```python
from build123d import *

# Parameters (mm, degrees)
PIN_DRAWING_W       = 0.636
PIN_DRAWING_H       = 0.636
BOSS_EXTRUDE1_DEPTH = 2.54


with BuildPart() as part:
    # pin_drawing → Boss-Extrude1 (new body)
    with BuildSketch(Plane.XY):
        Polygon((0, 2.146446609), (0, 0.353553391), (0.353553391, 0), (0, -0.353553391), (0, -2.146446609), (0.353553391, -2.5), (2.187446609, -2.5), (2.541, -2.146446609), (2.541, -0.353553391), (2.187446609, 0), (2.541, 0.353553391), (2.541, 2.146446609), (2.187446609, 2.5), (2.541, 2.853553391), (2.541, 4.646446609), (2.187446609, 5), (0.353553391, 5), (0, 4.646446609), (0, 2.853553391), (0.353553391, 2.5), align=None)
        with Locations((1.2705, -1.25)):
            Rectangle(PIN_DRAWING_W, PIN_DRAWING_H, mode=Mode.SUBTRACT)
        with Locations((1.2705, 1.25)):
            Rectangle(PIN_DRAWING_W, PIN_DRAWING_H, mode=Mode.SUBTRACT)
        with Locations((1.2705, 3.75)):
            Rectangle(PIN_DRAWING_W, PIN_DRAWING_H, mode=Mode.SUBTRACT)
    extrude(amount=BOSS_EXTRUDE1_DEPTH)


solid = part.part
```
Here's how the part is built. I have some questions about the finished solid (model axes, mm). Round coordinates to 2 decimals unless told otherwise and drop trailing zeros. Loops run counter-clockwise (first coordinate to the right, second up) from the corner with the lowest first, then second, coordinate; pieces in that order, holes last.
1. Will this pin go through, and if not, where does the flat tip stop? pin 1 (0.5 mm diameter, centred on y = -1.5, z = 1, fed in from -X).
Answers:
pin 1: stops at x = 0
2. Suppose I cut it at A-A, the plane x = 1.3. Please give me the cut outline in (y, z).
Answers:
outline: (-2.5, 0) - (-1.57, 0) - (-1.57, 2.54) - (-2.5, 2.54) - close; (-0.93, 0) - (0.93, 0) - (0.93, 2.54) - (-0.93, 2.54) - close; (1.57, 0) - (3.43, 0) - (3.43, 2.54) - (1.57, 2.54) - close; (4.07, 0) - (5, 0) - (5, 2.54) - (4.07, 2.54) - close
3. If I drill on probe 1 along Y at (x, z) = (1.25, 2.05); probe 2 along X at (y, z) = (-1.25, 1.2); probe 3 along Y at (x, z) = (2.45, 1.75), over which ranges is the centre line in solid material (lowest first)?
Answers:
probe 1: y = -2.5 to -1.57, -0.93 to 0.93, 1.57 to 3.43, 4.07 to 5
probe 2: x = 0 to 0.95, 1.59 to 2.54
probe 3: y = -2.24 to -0.26, 0.26 to 2.24, 2.76 to 4.74
4. Suppose I cut it at C-C, the plane y = 2.75. Please give me the cut outline in (x, z).
Answers:
outline: (0.1, 0) - (2.44, 0) - (2.44, 2.54) - (0.1, 2.54) - close
5. Suppose I cut it at B-B, the plane z = 2.2. Give the number of separate pieces and of enclosed holes in the cut face, and give its area (3 significant figures).
Answers:
separate pieces: 1
enclosed holes: 3
area: 17.1 mm2
